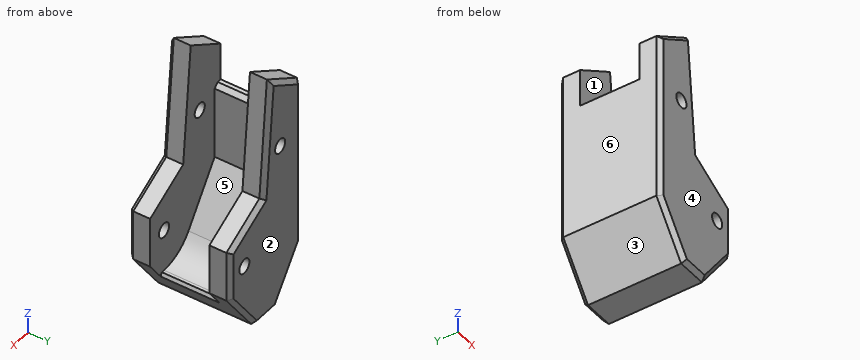
from build123d import *

# Parameters (mm, degrees)
PAD009_DEPTH    = 14
SKETCH008_R     = 1.7
PAD008_DEPTH    = 24
CHAMFER005_SIZE = 1


with BuildPart() as pad009:
    # Sketch009 → Pad009 (new body)
    with BuildSketch(Plane(origin=(0, 33, 0), x_dir=(-1, 0, 0), z_dir=(0, 1, 0))):
        with BuildLine():
            ThreePointArc((89.000023, -13), (93.632628, -11.86221), (97.21105, -8.707771))
            Line((97.21105, -8.707771), (106, 3.935782))
            Line((106, 3.935782), (106, 22))
            Line((106, 22), (112.578117, 22))
            Line((112.578117, 22), (112.578117, 42.659393))
            Line((112.578117, 42.659393), (77.159645, 42.659393))
            Line((77.159645, 42.659393), (77.159645, -13))
            Line((77.159645, -13), (89.000023, -13))
        make_face()
    extrude(amount=-PAD009_DEPTH)


with BuildPart() as foot:
    # Sketch008 → Pad008 (new body)
    with BuildSketch(Plane(origin=(0, 14, 0), x_dir=(-1, 0, 0), z_dir=(0, 1, 0))):
        Polygon((84.351819, 2.970513), (95.443832, 9.10709), (97.968148, 37.19022), (108, 30.921623), (108, -9), (99.675909, -20.407844), (92.675909, -20.407844), (84.351819, -9), align=None)
        with Locations((101, 19)):
            Circle(SKETCH008_R, mode=Mode.SUBTRACT)
        with Locations((89, -3)):
            Circle(SKETCH008_R, mode=Mode.SUBTRACT)
    extrude(amount=PAD008_DEPTH)

    # Cut014: cut Pad009
    add(pad009.part, mode=Mode.SUBTRACT)

    # Chamfer005
    chamfer005_edges = [foot.edges().sort_by_distance(p)[0] for p in [
        (-89.897825, 14, 6.038802),
        (-96.70599, 14, 23.148655),
        (-102.984074, 14, 34.055922),
        (-108, 14, 10.960812),
        (-103.837955, 14, -14.703922),
        (-96.175909, 14, -20.407844),
        (-88.513864, 14, -14.703922),
        (-84.351819, 14, -3.014744),
        (-108, 38, 10.960812),
        (-103.837955, 38, -14.703922),
        (-96.175909, 38, -20.407844),
        (-87.270544, 26, -13),
        (-88.513864, 38, -14.703922),
        (-106, 26, 22),
        (-89.897825, 38, 6.038802),
        (-96.70599, 38, 23.148655),
        (-102.984074, 38, 34.055922),
        (-84.351819, 38, -3.014744),
    ]]
    chamfer(chamfer005_edges, length=CHAMFER005_SIZE)


solid = foot.part
Geometry check sheet. Reference: the model listing, model coordinates, mm. Face numbers are marked on the shaded views. A direction names the side the tool comes from. Round coordinates to 2 decimals unless told otherwise and drop trailing zeros. Order: outer loops, then holes, each group sorted by start corner. A loop starts at its lowest first (then second) coordinate and runs counter-clockwise, first axis right, second up. Notation, with made-up numbers: (56, 84.5) -> (77, 84.5) arc R23 ccw to (77, 119.5) -> close; hole circle Ø6 at (58, 86.25). An arc over 180 degrees is marked (long way). Use one line per item in the form item = value.
1. Cross-section at C-C, the plane z = 19. Enter the section's corners in (x, y).
Working result:
outline = (-108, 15) -> (-107, 14) -> (-102.7, 14) -> (-102.7, 19) -> (-106, 19) -> (-106, 33) -> (-102.7, 33) -> (-102.7, 38) -> (-107, 38) -> (-108, 37) -> close; (-99.3, 14) -> (-97.34, 14) -> (-96.33, 15) -> (-96.33, 19) -> (-99.3, 19) -> close; (-99.3, 33) -> (-96.33, 33) -> (-96.33, 37) -> (-97.34, 38) -> (-99.3, 38) -> close
2. Go/stop test with flat-tipped pins: pin 1 (4 mm diameter, centred on x = -101, z = 19, fed in from -Y); pin 2 (3 mm diameter, centred on y = 25, z = -3.5, fed in from +X); pin 3 (0.5 mm diameter, centred on x = -107.5, y = 24.5, fed in from +Z); pin 4 (0.6 mm diameter, centred on x = -88.5, y = 25, fed in from +Z). Record where each tip stops, or that it passes through.
Working result:
pin_1 = 14
pin_2 = -99.79
pin_3 = 22
pin_4 = -13
3. Set-up check for the marked faces 5 and 6: record each of +Z, -Z, +X, -X, +Y, -Y from which the full face is reachable in a straight line by a thin tool's end or side.
Working result:
face_5 = +Z, +X
face_6 = +Z, -Z, -X, +Y, -Y
4. Cross-section at D-D, the plane y = 22.5. Enter the section's corners in (x, z), plus the area to 3 significant figures.
Working result:
outline = (-108, -9) -> (-99.68, -20.41) -> (-92.68, -20.41) -> (-87.86, -13.81) -> (-88.27, -13) -> (-89, -13) arc R10 cw to (-97.21, -8.71) -> (-106, 3.94) -> (-106, 21) -> (-107, 22) -> (-108, 22) -> close
area = 259 mm^2
5. Mould release check, pull along Y, two halves, no side actions. Record for the marked faces 1, 2, 3 and 4: pulls with the +Y half, pulls with the -Y half, needs draft (parallel to the pull), parting line crosses it, or undercut.
Working result:
face_1 = undercut
face_2 = pulls with the +Y half
face_3 = needs draft
face_4 = pulls with the -Y half
6. Cross-section at A-A, the plane y = 35.75. Enter the section's corners in (x, z).
Working result:
outline = (-108, -9) -> (-99.68, -20.41) -> (-92.68, -20.41) -> (-84.35, -9) -> (-84.35, 2.97) -> (-95.44, 9.11) -> (-97.97, 37.19) -> (-108, 30.92) -> close; hole circle Ø3.4 at (-101, 19); hole circle Ø3.4 at (-89, -3)
7. Scan lines: line 1 along X through (y, z) = (15.4, -3); line 2 along Y through (x, z) = (-102, 3); line 3 along X through (y, z) = (23.5, 16). Record each from-to range of solid material in increasing order. Write a range as from..to.
Working result:
line_1 = -108..-90.7, -87.3..-84.35
line_2 = 14..19, 33..38
line_3 = -108..-106
8. Cross-section at B-B, the plane x = -101. Enter the section's corners in (y, z).
Working result:
outline = (14, -16.9) -> (15, -18.59) -> (37, -18.59) -> (38, -16.9) -> (38, 17.3) -> (33, 17.3) -> (33, -3.26) -> (19, -3.26) -> (19, 17.3) -> (14, 17.3) -> close; (14, 20.7) -> (19, 20.7) -> (19, 35.3) -> (15, 35.3) -> (14, 34.12) -> close; (33, 20.7) -> (38, 20.7) -> (38, 34.12) -> (37, 35.3) -> (33, 35.3) -> close
